Could you check a few things on this model? Use its own coordinates, in mm. A direction names the side the tool comes from. Round coordinates to 2 decimals unless told otherwise and drop trailing zeros. Loops run counter-clockwise (first coordinate to the right, second up) from the corner with the lowest first, then second, coordinate; pieces in that order, holes last. Notation, with made-up numbers: (63.25, 23) -> (116.25, 23) arc R34 ccw to (116.25, 53) -> close; hole circle Ø11 at (57, 21). An arc over 180 degrees is marked (long way). Write each question's results on one line, items separated by ' | '. Start each with the question number.
1) Which directions (+Z, -Z, +X, -X, +Y, -Y) give clear straight access to the entire face, cutting with the end or side of a thin tool? Please do faces 3 (the flat face through (-66, -14, 39)), 4 (the cylindrical face through (-0.673, -104.996, 39.44)), 5 (the flat face through (57, -70, 39)), 6 (the cylindrical face through (53.118, -66.592, 20.176)).
2) Imagine slicing it at A-A, the plane y = -40. List the corners of the cut face in (x, z) for me, plus the area to 3 significant figures.
3) Imagine slicing it at B-B, the plane x = 0. List the corners of the cut face in (y, z) for me.
4) Imagine slicing it at D-D, the plane y = -59. List the corners of the cut face in (x, z) for me.
5) We'd pull the mould along Z, two halves only. Please class faces 1 (the conical face through (49.442, -27.014, 59.384)), 2 (the flat face through (45, -52.5, 39)): pulls with the +Z half, pulls with the -Z half, needs draft (parallel to the pull), parting line crosses it, or undercut.
6) If I drill on probe 1 along X at (y, z) = (-68, 42); probe 2 along Y at (x, z) = (42.5, 15.5); probe 3 along Y at (x, z) = (55, 38.5), over which ranges is the centre line in solid material (lowest first)?
7) Imagine slicing it at C-C, the plane z = 29. List the corners of the cut face in (x, y) for me, plus the area to 3 significant figures.
8) For P1, Ø12.5, axis at x = 49.12, z = 40, coming from the -Y side; P2, Ø12, axis at x = -58.5, z = 19.5, coming from the -Y side; P3, Ø5, axis at y = -67.5, z = 61, coming from the -X side; P4, Ø6, axis at x = 56, z = 27, coming from the +Y side, each with a flat end and sliding along its axis, tell me the tip position at first contact or that it passes through.
from build123d import *

# Parameters (mm, degrees)
F1_DEPTH       = 80
F3_D           = 8
F3_DEPTH       = 55
F3_CBORE_D     = 14
F3_CBORE_DEPTH = 6
F3_TIP         = 2.4034424761


# Not quite as in the source:
# - a feature of the source that left no trace in its solid (it failed there, or was rolled back) is left out


with BuildPart() as f1:
    # F0 (on Top) → F1 (new body)
    with BuildSketch(Plane.XY):
        with BuildLine():
            ThreePointArc((-31.6385840391, -14), (0, -3), (31.6385840391, -14))
            Line((31.6385840391, -14), (57, -14))
            Line((57, -14), (75, -14))
            Line((75, -14), (75, 0))
            Line((75, 0), (-75, 0))
            Line((-75, 0), (-75, -14))
            Line((-75, -14), (-57, -14))
            Line((-57, -14), (-31.6385840391, -14))
        make_face()
        with BuildLine():
            ThreePointArc((-41.2431812546, -84), (-50.5266061405, -47.0673185622), (-31.6385840391, -14))
            Line((-31.6385840391, -14), (-57, -14))
            Line((-57, -14), (-57, -84))
            Line((-57, -84), (-41.2431812546, -84))
        make_face()
        with BuildLine():
            ThreePointArc((0, -14), (27.748873851, -25.1902794182), (39.9718651053, -52.5))
            Line((39.9718651053, -52.5), (50.9779364039, -52.5))
            ThreePointArc((50.9779364039, -52.5), (45.5734008225, -31.1075309878), (31.6385840391, -14))
            Line((31.6385840391, -14), (0, -14))
        make_face()
        with BuildLine():
            ThreePointArc((-26.4575131106, -84), (-37.4165738677, -39.8578643763), (0, -14))
            Line((0, -14), (-31.6385840391, -14))
            ThreePointArc((-31.6385840391, -14), (-50.5266061405, -47.0673185622), (-41.2431812546, -84))
            Line((-41.2431812546, -84), (-26.4575131106, -84))
        make_face()
        with BuildLine():
            Line((57, -55.5), (50.9779364039, -55.5))
            ThreePointArc((50.9779364039, -55.5), (48.2622640947, -70.4849587338), (41.2431812546, -84))
            Line((41.2431812546, -84), (57, -84))
            Line((57, -84), (57, -55.5))
        make_face()
        with BuildLine():
            ThreePointArc((31.6385840391, -14), (45.5734008225, -31.1075309878), (50.9779364039, -52.5))
            Line((50.9779364039, -52.5), (57, -52.5))
            Line((57, -52.5), (57, -14))
            Line((57, -14), (31.6385840391, -14))
        make_face()
        with BuildLine():
            Line((41.2431812546, -84), (26.4575131106, -84))
            ThreePointArc((26.4575131106, -84), (0, -94), (-26.4575131106, -84))
            Line((-26.4575131106, -84), (-41.2431812546, -84))
            ThreePointArc((-41.2431812546, -84), (0, -105), (41.2431812546, -84))
        make_face()
        with BuildLine():
            Line((50.9779364039, -55.5), (39.9718651053, -55.5))
            ThreePointArc((39.9718651053, -55.5), (36.1424690986, -71.1383175213), (26.4575131106, -84))
            Line((26.4575131106, -84), (41.2431812546, -84))
            ThreePointArc((41.2431812546, -84), (48.2622640947, -70.4849587338), (50.9779364039, -55.5))
        make_face()
        with BuildLine():
            Line((-31.6385840391, -14), (0, -14))
            Line((0, -14), (31.6385840391, -14))
            ThreePointArc((31.6385840391, -14), (0, -3), (-31.6385840391, -14))
        make_face()
    extrude(amount=F1_DEPTH)

    # F3
    with Locations(Plane.XZ.offset(84)):
        with Locations((49.1215906273, 20), (49.1215906273, 40), (49.1215906273, 60)):
            CounterBoreHole(F3_D / 2, F3_CBORE_D / 2, F3_CBORE_DEPTH, depth=F3_DEPTH)
            with Locations((0, 0, -(F3_DEPTH + F3_TIP / 2))):  # 118° drill point
                Cone(0, F3_D / 2, F3_TIP, mode=Mode.SUBTRACT)


solid = f1.part
Checked values:
1) face 3: +Z, -Z, -X, -Y | face 4: +Z, -Z, -Y | face 5: +Z, -Z, +X, -Y | face 6: -Y
2) outline: (-57, 0) -> (-37.47, 0) -> (-37.47, 80) -> (-57, 80) -> close; (37.47, 0) -> (57, 0) -> (57, 80) -> (37.47, 80) -> close; hole circle Ø8 at (49.12, 20); hole circle Ø8 at (49.12, 40); hole circle Ø8 at (49.12, 60) | area: 2,970 mm^2
3) outline: (-105, 0) -> (-94, 0) -> (-94, 80) -> (-105, 80) -> close; (-14, 0) -> (0, 0) -> (0, 80) -> (-14, 80) -> close
4) outline: (-57, 0) -> (-39.69, 0) -> (-39.69, 80) -> (-57, 80) -> close; (39.69, 0) -> (57, 0) -> (57, 80) -> (39.69, 80) -> close; hole circle Ø8 at (49.12, 20); hole circle Ø8 at (49.12, 40); hole circle Ø8 at (49.12, 60)
5) face 1: undercut | face 2: needs draft
6) probe 1: -57 to -37.47, 37.47 to 45.66, 52.59 to 57 | probe 2: -84 to -55.5, -52.5 to 0 | probe 3: -78 to -55.5, -52.5 to 0
7) outline: (-75, -14) -> (-57, -14) -> (-57, -84) -> (-41.24, -84) arc R51 ccw to (41.24, -84) -> (57, -84) -> (57, -55.5) -> (39.97, -55.5) arc R40 cw (long way) to (39.97, -52.5) -> (57, -52.5) -> (57, -14) -> (75, -14) -> (75, 0) -> (-75, 0) -> close | area: 6,220 mm^2
8) P1: y = -78 | P2: y = -84 | P3: x = -57 | P4: y = 0
